from build123d import *

# Parameters (mm, degrees)
CROQUIS2_R                = 4.7625
SALIENTE_EXTRUIR1_DEPTH   = 24.5872
CHAFL_N1_SIZE             = 0.396875
CROQUIS4_R                = 2.4892
CLEARANCE_HOLE_DEPTH      = 25.5872
CLEARANCE_HOLE_DEPTH_BACK = 25.5872


with BuildPart() as part:
    # Croquis2 → Saliente-Extruir1 (new body, symmetric)
    with BuildSketch(Plane(origin=(0, 0, 0), x_dir=(1, 0, 0), z_dir=(0, 1, 0))):
        Circle(CROQUIS2_R)
    extrude(amount=SALIENTE_EXTRUIR1_DEPTH, both=True)

    # Chafl_n1
    chafl_n1_edges = [part.edges().sort_by_distance(p)[0] for p in [
        (-4.7625, -24.5872, 0),
        (-4.7625, 24.5872, 0),
    ]]
    chamfer(chafl_n1_edges, length=CHAFL_N1_SIZE)

    # Croquis4 → Clearance Hole (cut, two sides)
    with BuildSketch(Plane(origin=(0, 0, 0), x_dir=(1, 0, 0), z_dir=(0, 1, 0))) as clearance_hole_sk:
        Circle(CROQUIS4_R)
    extrude(amount=CLEARANCE_HOLE_DEPTH, mode=Mode.SUBTRACT)
    extrude(clearance_hole_sk.sketch, amount=-CLEARANCE_HOLE_DEPTH_BACK, mode=Mode.SUBTRACT)


solid = part.part
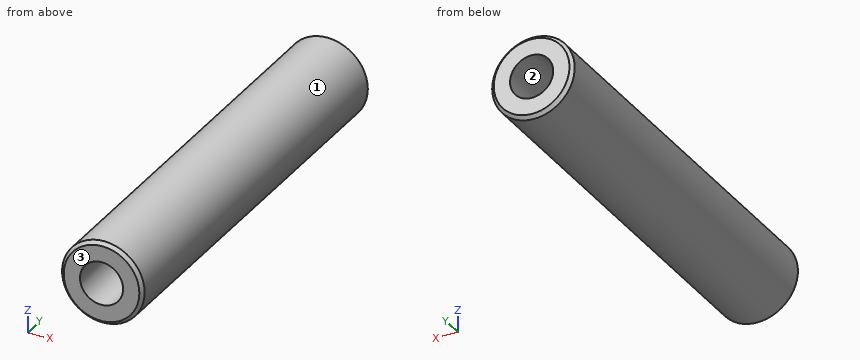
Read the model definition and answer for the solid it produces. Units are mm, in the model's axes. Face numbers are marked on the shaded views. Round coordinates to 2 decimals unless told otherwise and drop trailing zeros. Loops run counter-clockwise (first coordinate to the right, second up) from the corner with the lowest first, then second, coordinate; pieces in that order, holes last. Notation, with made-up numbers: (65, 33) - (120, 33) arc R35 cw to (120, 65) - close; hole circle Ø6 at (12, -35). An arc over 180 degrees is marked (long way). One line per question, with ' | ' between items. Start each with the question number.
Q1. Section C-C on y = 6.5 is taken. Give the vertices of the cut face in (x, z) (1 decimal), plus the area to 3 significant figures.
Q2. Flat-ended cylindrical pins translate along their axes: pin 1 (1.5 mm diameter, centred on x = -3.5, z = 4, fed in from +Y); pin 2 (3 mm diameter, centred on x = 2, y = 14.5, fed in from +Z); pin 3 (1 mm diameter, centred on x = -3.5, y = -12, fed in from -Z). Find the tip coordinate at first contact, or state that the pin passes through.
Q3. Section B-B on z = 0 is taken. Give the vertices of the cut face in (x, y), plus the area to 3 significant figures.
Q4. Find the intervals of material crossed by L1, parallel to Z at x = 0, y = -15; L2, parallel to X at y = -8.5, z = -0.5, in increasing order.
Q5. Section A-A on x = 0 is taken. Give the vertices of the cut face in (y, z), plus the area to 3 significant figures.
Q6. For a pull along Z with two mould halves and no side action, classify the marked faces 1, 2 and 3 as +Z half, -Z half, draft (parallel to the pull), parting line (faces both ways), or undercut.
Established:
1) outline: circle Ø9.5 at (0, 0); hole circle Ø5 at (0, 0) | area: 51.8 mm²
2) pin 1: y = 24.39 | pin 2: z = 4.74 | pin 3: z = -3.7
3) outline: (-4.76, -24.19) - (-4.37, -24.59) - (-2.49, -24.59) - (-2.49, 24.59) - (-4.37, 24.59) - (-4.76, 24.19) - close; (2.49, -24.59) - (4.37, -24.59) - (4.76, -24.19) - (4.76, 24.19) - (4.37, 24.59) - (2.49, 24.59) - close | area: 223 mm²
4) L1: -4.76 to -2.49, 2.49 to 4.76 | L2: -4.74 to -2.44, 2.44 to 4.74
5) outline: (-24.59, -4.37) - (-24.19, -4.76) - (24.19, -4.76) - (24.59, -4.37) - (24.59, -2.49) - (-24.59, -2.49) - close; (-24.59, 2.49) - (24.59, 2.49) - (24.59, 4.37) - (24.19, 4.76) - (-24.19, 4.76) - (-24.59, 4.37) - close | area: 223 mm²
6) face 1: parting line | face 2: undercut | face 3: draft
